from build123d import *

# Parameters (mm, degrees)
SKETCH1_W           = 33
SKETCH1_H           = 33
SKETCH1_W_2         = 31
SKETCH1_H_2         = 31
BOSS_EXTRUDE1_DEPTH = 3
SKETCH2_W           = 33
SKETCH2_H           = 33
BOSS_EXTRUDE2_DEPTH = 1
SKETCH3_R           = 6
CUT_EXTRUDE1_DEPTH  = 5
SKETCH4_R           = 8
BOSS_EXTRUDE3_DEPTH = 1


with BuildPart() as part:
    # Sketch1 → Boss-Extrude1 (new body)
    with BuildSketch(Plane(origin=(0, 0, 0), x_dir=(1, 0, 0), z_dir=(0, 1, 0))):
        Rectangle(SKETCH1_W, SKETCH1_H)
        Rectangle(SKETCH1_W_2, SKETCH1_H_2, mode=Mode.SUBTRACT)
    extrude(amount=BOSS_EXTRUDE1_DEPTH)

    # Sketch2 → Boss-Extrude2 (add)
    with BuildSketch(Plane(origin=(0, 3, 0), x_dir=(1, 0, 0), z_dir=(0, 1, 0))):
        Rectangle(SKETCH2_W, SKETCH2_H)
    extrude(amount=BOSS_EXTRUDE2_DEPTH)

    # Sketch3 → Cut-Extrude1 (cut, through all)
    with BuildSketch(Plane(origin=(0, 4, 0), x_dir=(1, 0, 0), z_dir=(0, 1, 0))):
        Circle(SKETCH3_R)
    extrude(amount=-CUT_EXTRUDE1_DEPTH, mode=Mode.SUBTRACT)

    # Sketch4 → Boss-Extrude3 (add)
    with BuildSketch(Plane.XZ.offset(-3)):
        Circle(SKETCH4_R)
    extrude(amount=BOSS_EXTRUDE3_DEPTH)


solid = part.part
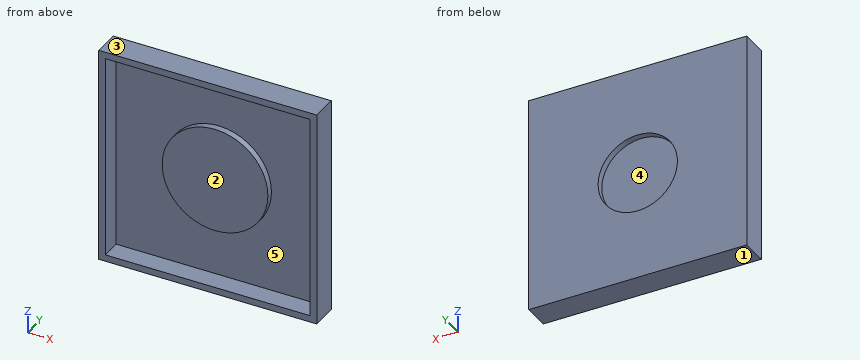
Geometry: final body of the model. Coordinates: model frame, mm. Face numbers are marked on the shaded views. A direction names the side the tool comes from. Give positions to 0.01 mm unless a question says otherwise; leave off trailing zeros. Order: outer loops, then holes, each group sorted by start corner. A loop starts at its lowest first (then second) coordinate and runs counter-clockwise, first axis right, second up. Notation, with made-up numbers: (-34, 14) -> (-1, 14) arc R24 ccw to (-1, 42) -> close; hole circle Ø7 at (-39.5, 11). An arc over 180 degrees is marked (long way). Answer as a JSON object with one key per item and string values.
Q1. Material intervals for probe 1 along Z at (x, y) = (0, 3.3); probe 2 along Z at (x, y) = (11, 1.95), sorted ascending.
Entries:
{"probe 1": "z = -16.5 to -6, 6 to 16.5", "probe 2": "z = -16.5 to -15.5, 15.5 to 16.5"}
Q2. Section A-A (y = 2.5). Output: boundary loops of the cut face in (x, z).
Entries:
{"outline": "(-16.5, -16.5) -> (16.5, -16.5) -> (16.5, 16.5) -> (-16.5, 16.5) -> close; circle Ø16 at (0, 0); hole (-15.5, -15.5) -> (15.5, -15.5) -> (15.5, 15.5) -> (-15.5, 15.5) -> close"}
Q3. Draft query along X for the marked faces 1 and 2. Return one class per face: released by +X, released by -X, zero draft, split by the parting line, or undercut.
Entries:
{"face 1": "zero draft", "face 2": "undercut"}
Q4. Section C-C (x = 0). Output: boundary loops of the cut face in (y, z), plus the area to 3 significant figures.
Entries:
{"outline": "(0, -16.5) -> (4, -16.5) -> (4, -6) -> (3, -6) -> (3, 6) -> (4, 6) -> (4, 16.5) -> (0, 16.5) -> (0, 15.5) -> (3, 15.5) -> (3, 8) -> (2, 8) -> (2, -8) -> (3, -8) -> (3, -15.5) -> (0, -15.5) -> close", "area": "43.0 mm^2"}
Q5. First-contact query: pin 1 (11 mm diameter, centred on x = 0, z = 0, fed in from -Y). Flat tip, straight axial feed; report the tip coordinate or a pass-through.
Entries:
{"pin 1": "stops at y = 2"}
Q6. Section B-B (z = 12.5). Output: boundary loops of the cut face in (x, y), plus the area to 3 significant figures.
Entries:
{"outline": "(-16.5, 0) -> (-15.5, 0) -> (-15.5, 3) -> (15.5, 3) -> (15.5, 0) -> (16.5, 0) -> (16.5, 4) -> (-16.5, 4) -> close", "area": "39.0 mm^2"}
Q7. Access query for the marked faces 3, 4 and 5. Directions: +Z, -Z, +X, -X, +Y, -Y. A direction counts if a zero-diameter tool reaches every point of the face in a straight line with its end or side. Return the directions, or none.
Entries:
{"face 3": "+Z, +X, -X, +Y, -Y", "face 4": "+Y", "face 5": "-Y"}
Q8. Section D-D (z = 0). Output: boundary loops of the cut face in (x, y), plus the area to 3 significant figures.
Entries:
{"outline": "(-16.5, 0) -> (-15.5, 0) -> (-15.5, 3) -> (-8, 3) -> (-8, 2) -> (8, 2) -> (8, 3) -> (15.5, 3) -> (15.5, 0) -> (16.5, 0) -> (16.5, 4) -> (6, 4) -> (6, 3) -> (-6, 3) -> (-6, 4) -> (-16.5, 4) -> close", "area": "43.0 mm^2"}
